The listing builds one solid part. Answer for the finished solid, in the listing's coordinates (mm). A direction names the side the tool comes from. Round coordinates to 2 decimals unless told otherwise and drop trailing zeros. Loops run counter-clockwise (first coordinate to the right, second up) from the corner with the lowest first, then second, coordinate; pieces in that order, holes last. Notation, with made-up numbers: M 30,85.25 L 79,85.25 A17 cw 79,90.25 Z; hole C 79.5,-13.75 d8. An arc over 180 degrees is marked long. Answer as a JSON object with one key per item and string values.
```python
from build123d import *

# Parameters (mm, degrees)
SKETCH1_R           = 63.5
BOSS_EXTRUDE1_DEPTH = 1.6
SKETCH3_R           = 1.75
CUT_EXTRUDE4_DEPTH  = 1.6
SKETCH2_R           = 1.5
CUT_EXTRUDE5_DEPTH  = 1.6
CUT_EXTRUDE6_DEPTH  = 10


with BuildPart() as part:
    # Sketch1 → Boss-Extrude1 (new body)
    with BuildSketch(Plane.XY):
        Circle(SKETCH1_R)
    extrude(amount=BOSS_EXTRUDE1_DEPTH)

    # Sketch3 → Cut-Extrude4 (cut)
    with BuildSketch(Plane(origin=(0, 0, 0), x_dir=(-1, 0, 0), z_dir=(0, 0, -1))):
        with Locations((-34.006305458, 36.654756705)):
            Circle(SKETCH3_R)
        with Locations((-49.354669589, 8.007283544)):
            Circle(SKETCH3_R)
    extrude(amount=-CUT_EXTRUDE4_DEPTH, mode=Mode.SUBTRACT)

    # Sketch2 → Cut-Extrude5 (cut)
    with BuildSketch(Plane(origin=(0, 0, 0), x_dir=(-1, 0, 0), z_dir=(0, 0, -1))):
        with Locations((0, 50)):
            Circle(SKETCH2_R)
        with Locations((43.301270189, -25)):
            Circle(SKETCH2_R)
        with Locations((-43.301270189, -25)):
            Circle(SKETCH2_R)
    extrude(amount=-CUT_EXTRUDE5_DEPTH, mode=Mode.SUBTRACT)

    # Sketch4 → Cut-Extrude6 (cut)
    with BuildSketch(Plane(origin=(0, 0, 0), x_dir=(-1, 0, 0), z_dir=(0, 0, -1))):
        with BuildLine():
            Line((-52.935522776, 11.911126581), (-44.12091565, 7.188553002))
            ThreePointArc((-44.12091565, 7.188553002), (-44.461118004, 5.385481223), (-45.773816402, 4.103440508))
            Line((-45.773816402, 4.103440508), (-54.588423529, 8.826014086))
            ThreePointArc((-54.588423529, 8.826014086), (-54.248221174, 10.629085865), (-52.935522776, 11.911126581))
        make_face()
        with BuildLine():
            Line((-39.240059397, 37.473487247), (-30.425452271, 32.750913668))
            ThreePointArc((-30.425452271, 32.750913668), (-29.112753873, 34.032954384), (-28.772551518, 35.836026163))
            Line((-28.772551518, 35.836026163), (-37.587158645, 40.558599742))
            ThreePointArc((-37.587158645, 40.558599742), (-38.899857043, 39.276559026), (-39.240059397, 37.473487247))
        make_face()
    extrude(amount=-CUT_EXTRUDE6_DEPTH, mode=Mode.SUBTRACT)


solid = part.part
```
Item 1: Which of the six approach directions +Z, -Z, +X, -X, +Y, -Y give full straight-line access (tool end or side, diameter ignored) to faces 1 (the face through (-1, 1, 1.6)), 2 (the face through (34.894, 35.145, 0.789))?
Values follow:
{"face 1": "+Z, +X, -X, +Y, -Y", "face 2": "+Z, -Z"}
Item 2: Straight lines are drawn through the part: line 1 (Y direction, x = 0, z = 1); line 2 (X direction, y = -24, z = 0.95); line 3 (Y direction, x = -44, z = 1.4). For each, find the intervals that lie inside material, in ascending order.
Values follow:
{"line 1": "-63.5 to 48.5, 51.5 to 63.5", "line 2": "-58.79 to -44.42, -42.18 to 42.18, 44.42 to 58.79", "line 3": "-45.78 to -26.33, -23.67 to 45.78"}
Item 3: Determine the mould class of faces 3 (the face through (48.59, 9.583, 0.789)), 4 (the face through (-1, 1, 0)), 5 (the face through (-13.77, -61.99, 0.79)) for opening direction Y: released by +Y, released by -Y, zero draft, split by the parting line, or undercut.
Values follow:
{"face 3": "undercut", "face 4": "zero draft", "face 5": "split by the parting line"}
Item 4: The part is cut by section C-C (y = -25). Give the vertices of the cut face in (x, z).
Values follow:
{"outline": "M -58.37,0 L -44.8,0 L -44.8,1.6 L -58.37,1.6 Z; M -41.8,0 L 41.8,0 L 41.8,1.6 L -41.8,1.6 Z; M 44.8,0 L 58.37,0 L 58.37,1.6 L 44.8,1.6 Z"}
Item 5: The part is cut by section B-B (z = 0.8). Give the vertices of the cut face in (x, y).
Values follow:
{"outline": "C 0,0 d127; hole C -43.3,-25 d3; hole C 0,50 d3; hole M 28.77,35.84 A3.05 ccw 30.43,32.75 L 39.24,37.47 A3.05 ccw 37.59,40.56 Z; hole C 43.3,-25 d3; hole M 44.12,7.19 A3.05 ccw 45.77,4.1 L 54.59,8.83 A3.05 ccw 52.94,11.91 Z"}
Item 6: The part is cut by section D-D (y = 50). Give the vertices of the cut face in (x, z), then the cut area to 3 significant figures.
Values follow:
{"outline": "M -39.14,0 L -1.5,0 L -1.5,1.6 L -39.14,1.6 Z; M 1.5,0 L 39.14,0 L 39.14,1.6 L 1.5,1.6 Z", "area": "120 mm^2"}
Item 7: The part is cut by section A-A (x = 0). Give the vertices of the cut face in (y, z).
Values follow:
{"outline": "M -63.5,0 L 48.5,0 L 48.5,1.6 L -63.5,1.6 Z; M 51.5,0 L 63.5,0 L 63.5,1.6 L 51.5,1.6 Z"}
Item 8: A flat-ended cylindrical pin translates along its axis: P1, Ø4, axis at x = 21, y = 13.5, coming from the -Z side. Find the tip coordinate at first contact, or state that the pin passes through.
Values follow:
{"P1": "z = 0"}
